Could you check a few things on this model? Use its own coordinates, in mm. Give positions to 0.01 mm unless a question says otherwise; leave off trailing zeros. Loops run counter-clockwise (first coordinate to the right, second up) from the corner with the lowest first, then second, coordinate; pieces in that order, holes last. Notation, with made-up numbers: M 75.25,46 L 129.25,46 A35 ccw 129.25,80 Z; hole C -24,14.5 d5. An arc over 180 degrees is marked long. Use a Markdown table: item, result. Add a question column.
1) Suppose I cut it at B-B on x = 0. List the corners of the cut face in (y, z) for me.
2) If I drill on line 1 along Z through (x, y) = (0, 1.5); line 2 along Z through (x, y) = (4, -2); line 3 along Z through (x, y) = (-0.75, 0.5), over which ranges is the centre line in solid material (lowest first)? Write a range as [from, to].
3) We'd pull the mould along X, two halves only. Please class faces 1 (the cylindrical face through (3, 0, 0)), 2 (the flat face through (0, 4, -4)), 3 (the cylindrical face through (1.08, 0.05, -4.88)): +X half, -X half, draft (parallel to the pull), parting line (faces both ways), or undercut.
4) Suppose I cut it at A-A on z = 0. List the corners of the cut face in (x, y) for me, and give its area (3 significant figures).
5) Will these pins go through, and if not, where does the flat tip stop? pin 1 Ø1 at (x, y) = (2, -1) entering from +Z; pin 2 Ø3 at (y, z) = (-2, -1.5) entering from -X; pin 3 Ø2 at (y, z) = (-2, 2) entering from -X; pin 4 Ø2 at (x, y) = (-4, 0) entering from +Z.
6) Suppose I cut it at C-C on y = 2.5. List the corners of the cut face in (x, z) for me.
Autodesk Inventor part; units mm, degrees
ref_plane "YZ Plane" through (0, 0, 0) normal (1, 0, 0) x (0, 1, 0)
ref_plane "XZ Plane" through (0, 0, 0) normal (0, 1, 0) x (-1, 0, 0)
ref_plane "XY Plane" through (0, 0, 0) normal (0, 0, 1) x (1, 0, 0)
sketch "Esboço1" plane through (0, 0, 0) normal (0, 0, 1) x (1, 0, 0)
  line L0 (-6, 0) -> (1, 0) construction
  line L1 (0, -5.6) -> (0, 5.6) construction
  line L2 (-5, 4) -> (-3, 4)
  line L3 (-3, 4) -> (-3, -4)
  line L4 (-3, -4) -> (-5, -4)
  line L5 (-5, -4) -> (-5, 4)
  point P0 (0, 0)
  dimension "d1" = 8
  dimension "d2" = 10
  dimension "d3" = 6
revolve "Revolução1" add sketch "Esboço1" angle 360 about axis through (0, -10, 0) along (0, 1, 0)
chamfer "Chanfro1" distance 0.5 angle 45 4 edges at (5, -4, 0) (3, -4, 0) (3, 4, 0) (5, 4, 0)
properties part number "GRJ-03-117" material "Latão YL"
Answer block:
| question | item | result |
|---|---|---|
| 1 | outline | M -4,-4.5 L -3.5,-5 L 3.5,-5 L 4,-4.5 L 4,-3.5 L 3.5,-3 L -3.5,-3 L -4,-3.5 Z; M -4,3.5 L -3.5,3 L 3.5,3 L 4,3.5 L 4,4.5 L 3.5,5 L -3.5,5 L -4,4.5 Z |
| 2 | line 1 | z = [-5, -3], [3, 5] |
| 2 | line 2 | z = [-3, 3] |
| 2 | line 3 | z = [-4.94, -2.9], [2.9, 4.94] |
| 3 | face 1 | undercut |
| 3 | face 2 | draft |
| 3 | face 3 | parting line |
| 4 | outline | M -5,-3.5 L -4.5,-4 L -3.5,-4 L -3,-3.5 L -3,3.5 L -3.5,4 L -4.5,4 L -5,3.5 Z; M 3,-3.5 L 3.5,-4 L 4.5,-4 L 5,-3.5 L 5,3.5 L 4.5,4 L 3.5,4 L 3,3.5 Z |
| 4 | area | 31.0 mm^2 |
| 5 | pin 1 | stops at z = 4.77 |
| 5 | pin 2 | stops at x = -5 |
| 5 | pin 3 | stops at x = -4.9 |
| 5 | pin 4 | stops at z = 4 |
| 6 | outline | C 0,0 d10; hole C 0,0 d6 |
